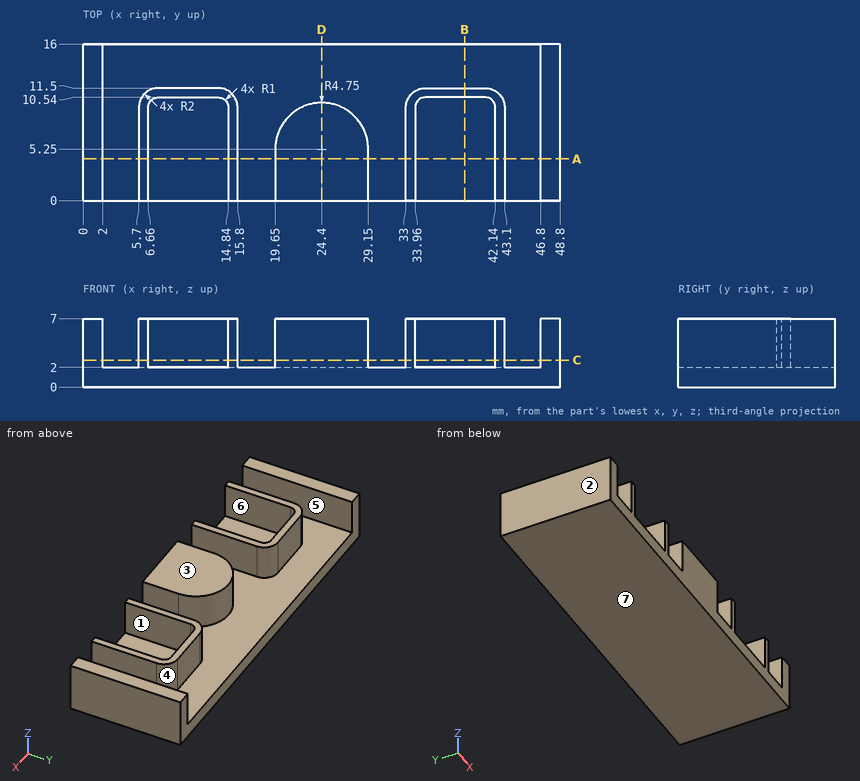
Design review of the part shown in the three views and the two pictorial views. Dimensions are in mm from the part's minimum x, y and z. A direction names the side the tool comes from. Coordinates: 2 decimals unless noted, no trailing zeros. Write each loop counter-clockwise with the first axis right and the second up, starting at its lowest first coordinate (ties: lowest second). Pieces come first, ordered by that corner, then holes. Notation, with made-up numbers: (61, -20.75) -> (108, -20.75) arc R26 ccw to (108, 14.25) -> close; hole circle Ø2 at (-4.5, 71.25). An arc over 180 degrees is marked (long way). Answer in a Markdown table with one row per item.
1. We need section C-C, the plane z = 2.75. Give the number of separate pieces and of enclosed holes in the cut face, and give its area (3 significant figures).
Answers below:
| item | result |
|---|---|
| separate pieces | 5 |
| enclosed holes | 0 |
| area | 207 mm^2 |
2. For the marked faces 4, 5, 6 and 7, list the 3-axis set-ups (+Z, -Z, +X, -X, +Y, -Y) from which the entire face can be reached by the end or side of a thin tool; tool diameter is ignored.
Answers below:
| item | result |
|---|---|
| face 4 | +Z, +Y |
| face 5 | +Z, +Y, -Y |
| face 6 | +Z, -Y |
| face 7 | -Z, +X, -X, +Y, -Y |
3. We need section A-A, the plane y = 4.25. State the section outline as (x, z) points, and give its area (3 significant figures).
Answers below:
| item | result |
|---|---|
| outline | (0, 0) -> (48.8, 0) -> (48.8, 7) -> (46.8, 7) -> (46.8, 2) -> (43.1, 2) -> (43.1, 7) -> (42.14, 7) -> (42.14, 2) -> (33.96, 2) -> (33.96, 7) -> (33, 7) -> (33, 2) -> (29.15, 2) -> (29.15, 7) -> (19.65, 7) -> (19.65, 2) -> (15.8, 2) -> (15.8, 7) -> (14.84, 7) -> (14.84, 2) -> (6.66, 2) -> (6.66, 7) -> (5.7, 7) -> (5.7, 2) -> (2, 2) -> (2, 7) -> (0, 7) -> close |
| area | 184 mm^2 |
4. We need section B-B, the plane x = 39. State the section outline as (y, z) points, and give its area (3 significant figures).
Answers below:
| item | result |
|---|---|
| outline | (0, 0) -> (16, 0) -> (16, 2) -> (11.5, 2) -> (11.5, 7) -> (10.54, 7) -> (10.54, 2) -> (0, 2) -> close |
| area | 36.8 mm^2 |
5. Clearance check with flat-ended pins moving along their axes: pin 1 Ø1.5 at (x, z) = (37, 4.5) entering from +Y; pin 2 Ø2.5 at (x, z) = (37, 4.5) entering from -Y. State where each tip first meets the part, or that it passes through.
Answers below:
| item | result |
|---|---|
| pin 1 | stops at y = 11.5 |
| pin 2 | stops at y = 10.54 |
6. Draft analysis for pull direction X (two halves, no side actions). For the marked faces 1, 2 and 3, state which applies: +X half, -X half, draft (parallel to the pull), parting line (faces both ways), or undercut.
Answers below:
| item | result |
|---|---|
| face 1 | undercut |
| face 2 | -X half |
| face 3 | draft |
7. We need section D-D, the plane x = 24.4. State the section outline as (y, z) points.
Answers below:
| item | result |
|---|---|
| outline | (0, 0) -> (16, 0) -> (16, 2) -> (10, 2) -> (10, 7) -> (0, 7) -> close |
8. Wall thickness on probe 1 along X at (y, z) = (10.25, 2.75); probe 2 along X at (y, z) = (11.25, 4); probe 3 along X at (y, z) = (15.25, 6): over which ranges is each line inside the solid? List them lowest first. Write a range as [from, to].
Answers below:
| item | result |
|---|---|
| probe 1 | x = [0, 2], [5.85, 6.96], [14.54, 15.65], [33.15, 34.26], [41.84, 42.95], [46.8, 48.8] |
| probe 2 | x = [0, 2], [6.73, 14.77], [34.03, 42.07], [46.8, 48.8] |
| probe 3 | x = [0, 2], [46.8, 48.8] |
